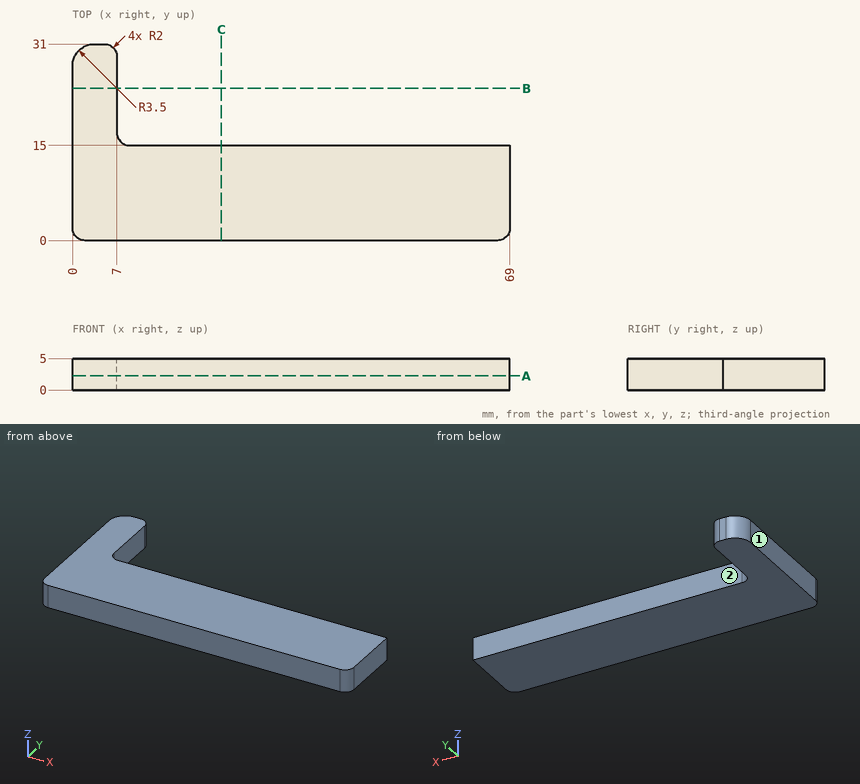
Design review of the part shown in the three views and the two pictorial views. Dimensions are in mm from the part's minimum x, y and z. A direction names the side the tool comes from. Round coordinates to 2 decimals unless told otherwise and drop trailing zeros. Write each loop counter-clockwise with the first axis right and the second up, starting at its lowest first coordinate (ties: lowest second). Pieces come first, ordered by that corner, then holes.
Item 1: For the marked faces 1 and 2, list the 3-axis set-ups (+Z, -Z, +X, -X, +Y, -Y) from which the entire face can be reached by the end or side of a thin tool; tool diameter is ignored.
Item 2: For probe 1 along X at (y, z) = (17.5, 0.85); probe 2 along Y at (x, z) = (24.5, 0.35); probe 3 along Y at (x, z) = (6, 2.45), list the stretches that pass through material, from the lowest coordinate up.
Item 3: We need section A-A on z = 2.25. Write out the cut boundary in (x, y), and give its area (3 significant figures).
Item 4: Clearance check with flat-ended pins moving along their axes: pin 1 Ø2.5 at (y, z) = (21, 2.5) entering from +X; pin 2 Ø3 at (x, z) = (31, 1) entering from +Y. State where each tip first meets the part, or that it passes through.
Item 5: We need section B-B on y = 24. Write out the cut boundary in (x, z), and give its area (3 significant figures).
Item 6: We need section C-C on x = 23.5. Write out the cut boundary in (y, z), and give its area (3 significant figures).
Returned:
1. face 1: +Z, -Z, -X, +Y, -Y
1. face 2: +Z, -Z, +X, +Y
2. probe 1: x = 0 to 7
2. probe 2: y = 0 to 15
2. probe 3: y = 0 to 30.73
3. outline: (0, 2) arc R2 ccw to (2, 0) - (67, 0) arc R2 ccw to (69, 2) - (69, 15) - (9, 15) arc R2 cw to (7, 17) - (7, 29) arc R2 ccw to (5, 31) - (3.5, 31) arc R3.5 ccw to (0, 27.5) - close
3. area: 1,140 mm2
4. pin 1: stops at x = 7
4. pin 2: stops at y = 15
5. outline: (0, 0) - (7, 0) - (7, 5) - (0, 5) - close
5. area: 35.0 mm2
6. outline: (0, 0) - (15, 0) - (15, 5) - (0, 5) - close
6. area: 75.0 mm2
